from build123d import *

# Parameters (mm, degrees)
SKETCH1_W           = 15.875
SKETCH1_H           = 9.525
BOSS_EXTRUDE1_DEPTH = 9.525
SKETCH2_W           = 9.525
SKETCH2_H           = 3.175
CUT_EXTRUDE1_DEPTH  = 12.7
SKETCH3_R           = 1.27
CUT_EXTRUDE2_DEPTH  = 9.525
SKETCH4_R           = 1.4605
CUT_EXTRUDE3_DEPTH  = 3.175


with BuildPart() as part:
    # Sketch1 → Boss-Extrude1 (new body)
    with BuildSketch(Plane(origin=(0, 0, 0), x_dir=(1, 0, 0), z_dir=(0, 1, 0))):
        Rectangle(SKETCH1_W, SKETCH1_H)
    extrude(amount=BOSS_EXTRUDE1_DEPTH)

    # Sketch2 → Cut-Extrude1 (cut)
    with BuildSketch(Plane.ZY.offset(7.9375)):
        with Locations((0, 4.7625)):
            Rectangle(SKETCH2_W, SKETCH2_H)
    extrude(amount=-CUT_EXTRUDE1_DEPTH, mode=Mode.SUBTRACT)

    # Sketch3 → Cut-Extrude2 (cut)
    with BuildSketch(Plane.XZ):
        with Locations(Location((-4.3815, 0, 0), (0, 0, 270))):
            Circle(SKETCH3_R)
    extrude(amount=-CUT_EXTRUDE2_DEPTH, mode=Mode.SUBTRACT)

    # Sketch4 → Cut-Extrude3 (cut)
    with BuildSketch(Plane.ZY.offset(-4.7625)):
        with Locations((0, 4.7625)):
            Circle(SKETCH4_R)
    extrude(amount=-CUT_EXTRUDE3_DEPTH, mode=Mode.SUBTRACT)


solid = part.part
The listing builds one solid part. Answer for the finished solid, in the listing's coordinates (mm). A direction names the side the tool comes from. Round coordinates to 2 decimals unless told otherwise and drop trailing zeros. Order: outer loops, then holes, each group sorted by start corner. A loop starts at its lowest first (then second) coordinate and runs counter-clockwise, first axis right, second up. Notation, with made-up numbers: M 56,64 L 86,64 A13 ccw 86,81 Z; hole C -17,54.25 d7. An arc over 180 degrees is marked long. Answer in a Markdown table with one row per item. Add a question column.
1) Determine the mould class of faces 1 (the face through (0, 7, -4.762)), 2 (the face through (6.328, 5.75, -1.076)), 3 (the face through (4.762, 6.196, -1.125)) for opening direction Z: pulls with the +Z half, pulls with the -Z half, needs draft (parallel to the pull), parting line crosses it, or undercut.
2) Consider line 1 along Y through (x, z) = (3.75, 1.25) (3 decimals); line 2 along Y through (x, z) = (7.25, 0) (3 decimals); line 3 along X through (y, z) = (7.45, 0). Determine where each line is inside the solid, lowest interval first. Write a range as from..to.
3) The part is cut by section C-C on y = 5.5. Determine the outline of the cut face in (x, z).
4) The part is cut by section A-A on z = 0. Count the separate pieces of the cut face and the enclosed holes in it, plus the area to 3 significant figures.
5) Which of the six approach directions +Z, -Z, +X, -X, +Y, -Y give full straight-line access (tool end or side, diameter ignored) to faces 4 (the face through (-2, 3.175, 0)), 5 (the face through (0, 9.525, 0))?
6) Flat-ended cylindrical pins translate along their axes: pin 1 Ø2.5 at (y, z) = (4.76, 0) entering from -X; pin 2 Ø1.6 at (y, z) = (5.5, 0) entering from -X. Find the tip coordinate at first contact, or state that the pin passes through.
Findings below:
| question | item | result |
|---|---|---|
| 1 | face 1 | pulls with the -Z half |
| 1 | face 2 | undercut |
| 1 | face 3 | needs draft |
| 2 | line 1 | y = 0..3.175, 6.35..9.525 |
| 2 | line 2 | y = 0..3.302, 6.223..9.525 |
| 2 | line 3 | x = -7.94..-5.65, -3.11..7.94 |
| 3 | outline | M 4.76,-4.76 L 7.94,-4.76 L 7.94,-1.26 L 4.76,-1.26 Z; M 4.76,1.26 L 7.94,1.26 L 7.94,4.76 L 4.76,4.76 Z |
| 4 | separate pieces | 4 |
| 4 | enclosed holes | 0 |
| 4 | area | 85.5 mm² |
| 5 | face 4 | +Z, -Z, -X |
| 5 | face 5 | +Z, -Z, +X, -X, +Y |
| 6 | pin 1 | passes through |
| 6 | pin 2 | stops at x = 4.76 |
